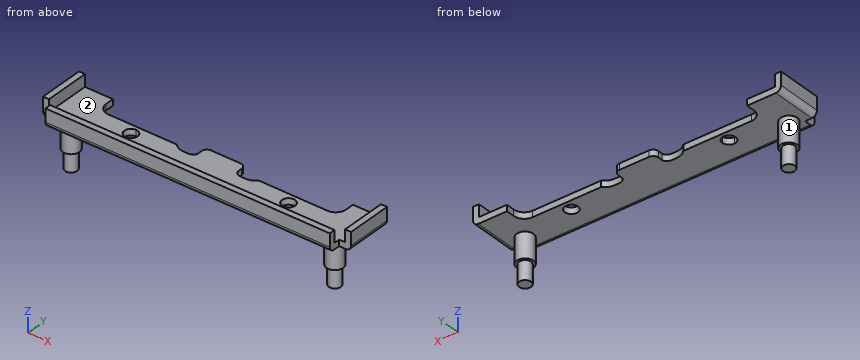
```python
from build123d import *

# Parameters (mm, degrees)
F0_R     = 2.01295
F0_R_2   = 1.44145
F1_DEPTH = 6.096
F2_DEPTH = 4.5466
F3_R     = 1.5875
F3_W     = 53.2003
F3_H     = 1.4478
F3_W_2   = 12.7762
F3_W_3   = 1.4478
F3_H_2   = 10.922
F3_W_4   = 2.4765
F4_DEPTH = 1.4732
F5_DEPTH = 4.3815
F6_R     = 1.27


with BuildPart() as f1:
    # F0 (on Top) → F1 (new body)
    with BuildSketch(Plane.XY):
        Circle(F0_R)
        Circle(F0_R_2, mode=Mode.SUBTRACT)
        Circle(F0_R_2)
    extrude(amount=F1_DEPTH)

    # F0 (on Top) → F2, piece 2 (join)
    with BuildSketch(Plane.XY):
        Circle(F0_R_2)
    extrude(amount=-F2_DEPTH)



with BuildPart() as f1b:
    # F0 (on Top) → F1, piece 2 (new body)
    with BuildSketch(Plane.XY):
        with BuildLine():
            ThreePointArc((65.51295, 0), (63.5, 2.01295), (61.48705, 0))
            ThreePointArc((61.48705, 0), (63.5, -2.01295), (65.51295, 0))
        make_face()
        with BuildLine():
            ThreePointArc((64.94145, 0), (63.5, -1.44145), (62.05855, 0))
            ThreePointArc((62.05855, 0), (63.5, 1.44145), (64.94145, 0))
        make_face(mode=Mode.SUBTRACT)
        with BuildLine():
            ThreePointArc((64.94145, 0), (63.5, 1.44145), (62.05855, 0))
            ThreePointArc((62.05855, 0), (63.5, -1.44145), (64.94145, 0))
        make_face()
    extrude(amount=F1_DEPTH)

    # F0 (on Top) → F2 (join)
    with BuildSketch(Plane.XY):
        with BuildLine():
            ThreePointArc((64.94145, 0), (63.5, 1.44145), (62.05855, 0))
            ThreePointArc((62.05855, 0), (63.5, -1.44145), (64.94145, 0))
        make_face()
    extrude(amount=-F2_DEPTH)


with BuildPart() as f1_1:
    add(f1.part)

    add(f1b.part)  # F4 merges F1b
    # F3 (on face) → F4 (join)
    with BuildSketch(Plane.XY.offset(6.096)):
        with BuildLine():
            Line((12.7762, -3.22072), (65.9765, -3.22072))
            Line((65.9765, -3.22072), (65.9765, -1.81102))
            Line((65.9765, -1.81102), (67.3862, -1.81102))
            Line((67.3862, -1.81102), (67.3862, 9.11098))
            Line((67.3862, 9.11098), (60.6679, 9.11098))
            Line((60.6679, 9.11098), (60.6679, 7.05358))
            ThreePointArc((60.6679, 7.05358), (59.9239512242, 5.2575287758), (58.1279, 4.51358))
            Line((58.1279, 4.51358), (48.4759, 4.51358))
            Line((48.4759, 4.51358), (41.656, 4.51358))
            add(Edge.make_bspline(
                [(41.656, 4.51358), (41.2915210924, 4.1758145401), (40.5551891723, 3.4567511883), (38.111648117, 3.3607328563), (37.2421413327, 3.55540528), (36.6106444724, 4.1422323132), (36.576, 4.51358)],
                knots=[0, 0, 0, 0, 0.2581839456, 0.5779890319, 0.781834691, 1, 1, 1, 1], degree=3))
            Line((36.576, 4.51358), (36.576, 5.68198))
            ThreePointArc((36.576, 5.68198), (36.2040256121, 6.5800056121), (35.306, 6.95198))
            Line((35.306, 6.95198), (31.75, 6.95198))
            Line((31.75, 6.95198), (28.194, 6.95198))
            ThreePointArc((28.194, 6.95198), (27.2959743879, 6.5800056121), (26.924, 5.68198))
            Line((26.924, 5.68198), (26.924, 4.51358))
            add(Edge.make_bspline(
                [(21.844, 4.51358), (22.2084789076, 4.1758145401), (22.9448108277, 3.4567511883), (25.388351883, 3.3607328563), (26.2578586673, 3.55540528), (26.8893555276, 4.1422323132), (26.924, 4.51358)],
                knots=[0, 0, 0, 0, 0.2581839456, 0.5779890319, 0.781834691, 1, 1, 1, 1], degree=3))
            Line((21.844, 4.51358), (12.7762, 4.51358))
            Line((12.7762, 4.51358), (12.7762, 3.64998))
            ThreePointArc((12.7762, 3.64998), (13.8987320151, 3.1850120151), (14.3637, 2.06248))
            ThreePointArc((14.3637, 2.06248), (13.8987320151, 0.9399479849), (12.7762, 0.47498))
            Line((12.7762, 0.47498), (12.7762, -3.22072))
        make_face()
        with Locations((50.7238, 2.06248)):
            Circle(F3_R, mode=Mode.SUBTRACT)
        with BuildLine():
            Line((0, -3.22072), (12.7762, -3.22072))
            Line((12.7762, -3.22072), (12.7762, 0.47498))
            ThreePointArc((12.7762, 0.47498), (11.1887, 2.06248), (12.7762, 3.64998))
            Line((12.7762, 3.64998), (12.7762, 4.51358))
            Line((12.7762, 4.51358), (5.3721, 4.51358))
            ThreePointArc((5.3721, 4.51358), (3.5760487758, 5.2575287758), (2.8321, 7.05358))
            Line((2.8321, 7.05358), (2.8321, 9.11098))
            Line((2.8321, 9.11098), (-3.8862, 9.11098))
            Line((-3.8862, 9.11098), (-3.8862, -1.81102))
            Line((-3.8862, -1.81102), (-2.4765, -1.81102))
            Line((-2.4765, -1.81102), (-2.4765, -3.22072))
            Line((-2.4765, -3.22072), (0, -3.22072))
        make_face()
        with BuildLine():
            ThreePointArc((2.01295, 0), (1.4233705952, -1.4233705952), (0, -2.01295))
            ThreePointArc((0, -2.01295), (-1.4233705952, 1.4233705952), (2.01295, 0))
        make_face(mode=Mode.SUBTRACT)
        with Locations((39.37635, -3.94462)):
            Rectangle(F3_W, F3_H)
        with Locations((6.3881, -3.94462)):
            Rectangle(F3_W_2, F3_H)
        with Locations((68.1101, 3.64998)):
            Rectangle(F3_W_3, F3_H_2)
        with Locations((-4.6101, 3.64998)):
            Rectangle(F3_W_3, F3_H_2)
        with BuildLine():
            ThreePointArc((2.01295, 0), (-1.4233705952, 1.4233705952), (0, -2.01295))
            ThreePointArc((0, -2.01295), (1.4233705952, -1.4233705952), (2.01295, 0))
        make_face()
        with Locations((-1.23825, -3.94462)):
            Rectangle(F3_W_4, F3_H)
    extrude(amount=F4_DEPTH)

    # F3 (on face) → F5 (join)
    with BuildSketch(Plane.XY.offset(6.096)):
        with Locations((-4.6101, 3.64998)):
            Rectangle(F3_W_3, F3_H_2)
        with Locations((6.3881, -3.94462)):
            Rectangle(F3_W_2, F3_H)
        with Locations((39.37635, -3.94462)):
            Rectangle(F3_W, F3_H)
        with Locations((68.1101, 3.64998)):
            Rectangle(F3_W_3, F3_H_2)
        with Locations((-1.23825, -3.94462)):
            Rectangle(F3_W_4, F3_H)
    extrude(amount=F5_DEPTH)

    # F6
    f6_edges = [f1_1.edges().sort_by_distance(p)[0] for p in [
        (-5.334, 3.64998, 6.096),
        (31.75, -4.66852, 6.096),
        (68.834, 3.64998, 6.096),
    ]]
    fillet(f6_edges, radius=F6_R)


solid = f1_1.part
```
Build history of the part. All positions in model axes, mm. Face numbers are marked on the shaded views. A direction names the side the tool comes from. Round coordinates to 2 decimals unless told otherwise and drop trailing zeros. Loops run counter-clockwise (first coordinate to the right, second up) from the corner with the lowest first, then second, coordinate; pieces in that order, holes last.
Item 1: Which spindle directions (+Z, -Z, +X, -X, +Y, -Y) get a long thin tool onto all of the face, cutting with end or side? Do the marked faces 1 and 2. Say none if no direction does.
Item 2: Drill centre lines: line 1 along X through (y, z) = (3.75, 9.5); line 2 along Z through (x, y) = (64, 3); line 3 along Y through (x, z) = (4, 7.75). Where is each one in solid material? Low to high.
Item 3: Saw through at D-D (z = 2). List the corners of the cut face in (x, y), then the cut area to 3 significant figures.
Item 4: Saw through at B-B (x = 20). List the corners of the cut face in (y, z).
Item 5: Saw through at A-A (y = 2.75). List the corners of the cut face in (x, z).
Item 6: Saw through at C-C (z = -0.75). List the corners of the cut face in (x, y), then the cut area to 3 significant figures.
Item 7: Pin check, flat tips, straight feed: P1, Ø1.5, axis at y = 2, z = 4, coming from the +X side; P2, Ø1.4, axis at y = -3.5, z = 9.5, coming from the +X side; P3, Ø8, axis at x = 29.5, y = 5, coming from the -Z side; P4, Ø1.5, axis at x = 15, y = 6.5, coming from the -Z side. Stop position of each tip, or through.
Worked answers:
1. face 1: -Z
1. face 2: +Z, +Y
2. line 1: x = -5.33 to -3.89, 67.39 to 68.83
2. line 2: z = 6.1 to 7.57
2. line 3: y = -4.67 to -3.22
3. outline: circle Ø4.03 at (0, 0); circle Ø4.03 at (63.5, 0)
3. area: 25.5 mm2
4. outline: (-4.67, 7.37) arc R1.27 ccw to (-3.4, 6.1) - (4.51, 6.1) - (4.51, 7.57) - (-3.22, 7.57) - (-3.22, 10.48) - (-4.67, 10.48) - close
5. outline: (-5.33, 7.37) arc R1.27 ccw to (-4.06, 6.1) - (11.35, 6.1) - (11.35, 7.57) - (-3.89, 7.57) - (-3.89, 10.48) - (-5.33, 10.48) - close; (14.21, 6.1) - (49.29, 6.1) - (49.29, 7.57) - (14.21, 7.57) - close; (52.15, 6.1) - (67.56, 6.1) arc R1.27 ccw to (68.83, 7.37) - (68.83, 10.48) - (67.39, 10.48) - (67.39, 7.57) - (52.15, 7.57) - close
6. outline: circle Ø2.88 at (0, 0); circle Ø2.88 at (63.5, 0)
6. area: 13.1 mm2
7. P1: stops at x = 65.08
7. P2: stops at x = 65.98
7. P3: stops at z = 6.1
7. P4: passes through
